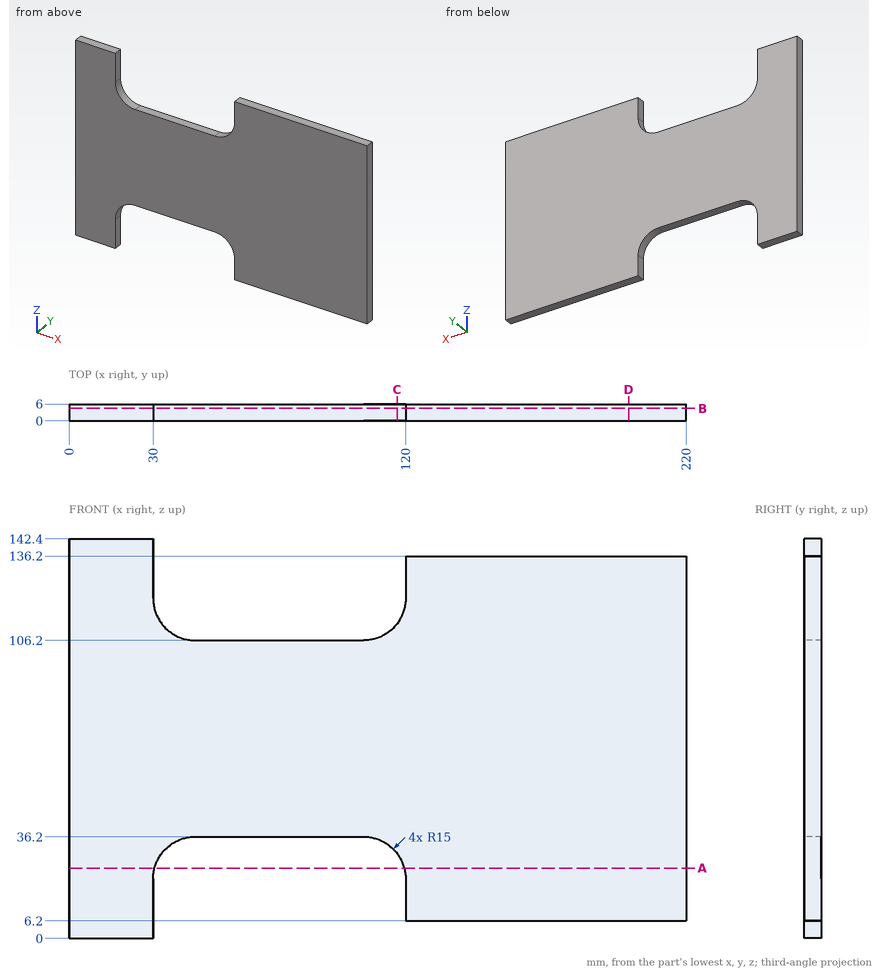
Geometry check sheet. Reference: drawing and pictorial views, mm from the part's lowest x, y, z. Round coordinates to 2 decimals unless told otherwise and drop trailing zeros. Write each loop counter-clockwise with the first axis right and the second up, starting at its lowest first coordinate (ties: lowest second). Pieces come first, ordered by that corner, then holes.
1. Section check C-C on x = 117. Enter the section's corners in (y, z), plus the area to 3 significant figures.
2. Scan lines: L1, parallel to X at y = 4.85, z = 11; L2, parallel to Z at x = 167.5, y = 5.55; L3, parallel to Z at x = 72, y = 2. Record each from-to range of solid material in increasing order.
3. Section check A-A on z = 25. Enter the section's corners in (x, y).
4. Section check D-D on x = 199.5. Enter the section's corners in (y, z).
5. Gauge pin test, flat ends, axial feed: P1, Ø3, axis at x = 61.5, y = 3.5, coming from the +Z side; P2, Ø1.8, axis at x = 169, y = 2.5, coming from the -Z side; P3, Ø2, axis at x = 156, y = 4.5, coming from the +Z side; P4, Ø1.5, axis at x = 123.5, z = 67, coming from the -Y side. Record the tip position at first contact, or that the pin passes through.
6. Section check B-B on y = 4.4. Enter the section's corners in (x, z), plus the area to 3 significant figures.
Answer:
1. outline: (0, 30.2) - (6, 30.2) - (6, 112.2) - (0, 112.2) - close
1. area: 492 mm2
2. L1: x = 0 to 30, 120 to 220
2. L2: z = 6.2 to 136.2
2. L3: z = 36.2 to 106.2
3. outline: (0, 0) - (30.49, 0) - (30.49, 6) - (0, 6) - close; (119.51, 0) - (220, 0) - (220, 6) - (119.51, 6) - close
4. outline: (0, 6.2) - (6, 6.2) - (6, 136.2) - (0, 136.2) - close
5. P1: stops at z = 106.2
5. P2: stops at z = 6.2
5. P3: stops at z = 136.2
5. P4: stops at y = 0
6. outline: (0, 0) - (30, 0) - (30, 21.2) arc R15 cw to (45, 36.2) - (105, 36.2) arc R15 cw to (120, 21.2) - (120, 6.2) - (220, 6.2) - (220, 136.2) - (120, 136.2) - (120, 121.2) arc R15 cw to (105, 106.2) - (45, 106.2) arc R15 cw to (30, 121.2) - (30, 142.4) - (0, 142.4) - close
6. area: 23,800 mm2
